Work out the finished part from the listing and answer in its coordinate system (mm). A direction names the side the tool comes from. Give positions to 0.01 mm unless a question says otherwise; leave off trailing zeros. Loops run counter-clockwise (first coordinate to the right, second up) from the corner with the lowest first, then second, coordinate; pieces in that order, holes last. Notation, with made-up numbers: M 15.5,-10.75 L 51.5,-10.75 A33 ccw 51.5,26.25 Z; hole C 29,64 d10. An arc over 180 degrees is marked long. Use a Markdown table: item, result.
```python
from build123d import *

# Parameters (mm, degrees)
SKETCH1_R                                    = 65
BOSS_EXTRUDE2_DEPTH                          = 30
SKETCH2_R                                    = 52.6
CUT_EXTRUDE1_DEPTH                           = 84
SKETCH4_R                                    = 52.6
BOSS_EXTRUDE3_DEPTH                          = 5
SKETCH5_W                                    = 16.2
SKETCH5_H                                    = 9.2
CUT_EXTRUDE2_DEPTH                           = 12
CUT_EXTRUDE3_DEPTH                           = 5.2
M6_CLEARANCE_HOLE1_D                         = 7
CUT_EXTRUDE4_START                           = -18
SKETCH11_R                                   = 65
CUT_EXTRUDE4_DEPTH                           = 18
SKETCH12_R                                   = 65
BOSS_EXTRUDE4_DEPTH                          = 5
CSK_FOR_M6_COUNTERSUNK_FLAT_HEAD_SCR_2_COUNT = 2
CSK_FOR_M6_COUNTERSUNK_FLAT_HEAD_SCR_2_PITCH = 35.355339059
CSK_FOR_M6_COUNTERSUNK_FLAT_HEAD_SCR_3_COUNT = 2
CSK_FOR_M6_COUNTERSUNK_FLAT_HEAD_SCR_3_PITCH = 50
CSK_FOR_M6_COUNTERSUNK_FLAT_HEAD_SCR_4_COUNT = 2
CSK_FOR_M6_COUNTERSUNK_FLAT_HEAD_SCR_4_PITCH = 50
CSK_FOR_M6_COUNTERSUNK_FLAT_HEAD_SCR_5_COUNT = 2
CSK_FOR_M6_COUNTERSUNK_FLAT_HEAD_SCR_5_PITCH = 35.355339059
CSK_FOR_M6_COUNTERSUNK_FLAT_HEAD_SCR_6_COUNT = 2
CSK_FOR_M6_COUNTERSUNK_FLAT_HEAD_SCR_6_PITCH = 35.355339059
CUT_EXTRUDE5_START                           = -3
SKETCH22_R                                   = 65
CUT_EXTRUDE5_DEPTH                           = 3


with BuildPart() as part:
    # Sketch1 → Boss-Extrude2 (new body)
    with BuildSketch(Plane(origin=(0, 0, 0), x_dir=(1, 0, 0), z_dir=(0, 1, 0))):
        with Locations(Location((0, 0, 0), (0, 0, 270))):
            Circle(SKETCH1_R)
    extrude(amount=BOSS_EXTRUDE2_DEPTH)

    # Sketch2 → Cut-Extrude1 (cut)
    with BuildSketch(Plane(origin=(0, 30, 0), x_dir=(1, 0, 0), z_dir=(0, 1, 0))):
        with Locations(Location((0, 0, 0), (0, 0, 270))):
            Circle(SKETCH2_R)
    extrude(amount=-CUT_EXTRUDE1_DEPTH, mode=Mode.SUBTRACT)

    # Sketch4 → Boss-Extrude3 (add)
    with BuildSketch(Plane(origin=(0, 30, 0), x_dir=(1, 0, 0), z_dir=(0, 1, 0))):
        with Locations(Location((0, 0, 0), (0, 0, 270))):
            Circle(SKETCH4_R)
    extrude(amount=-BOSS_EXTRUDE3_DEPTH)

    # Sketch5 → Cut-Extrude2 (cut)
    with BuildSketch(Plane.XZ):
        with Locations((-52.6, 0)):
            Rectangle(SKETCH5_W, SKETCH5_H)
        with Locations((52.6, 0)):
            Rectangle(SKETCH5_W, SKETCH5_H)
    extrude(amount=-CUT_EXTRUDE2_DEPTH, mode=Mode.SUBTRACT)

    # Sketch7 → Cut-Extrude3 (cut)
    with BuildSketch(Plane.XZ.offset(-12)):
        with BuildLine():
            Line((37.19381669, -37.19381669), (44.070308528, -44.070308528))
            ThreePointArc((44.070308528, -44.070308528), (57.580632973, -23.850679107), (62.324828018, 0))
            Line((62.324828018, 0), (52.6, 0))
            ThreePointArc((52.6, 0), (48.59606341, -20.129148542), (37.19381669, -37.19381669))
        make_face()
        with BuildLine():
            Line((-37.19381669, 37.19381669), (-44.070308528, 44.070308528))
            ThreePointArc((-44.070308528, 44.070308528), (-57.580632973, 23.850679107), (-62.324828018, 0))
            Line((-62.324828018, 0), (-52.6, 0))
            ThreePointArc((-52.6, 0), (-48.59606341, 20.129148542), (-37.19381669, 37.19381669))
        make_face()
    extrude(amount=CUT_EXTRUDE3_DEPTH, mode=Mode.SUBTRACT)

    # M6 Clearance Hole1 (through all)
    with Locations(Plane(origin=(0, 30, -25), x_dir=(0, 0, 1), z_dir=(0, 1, 0))):
        with Locations((0, 0), (25, -25), (25, 25), (50, 0)):
            Hole(M6_CLEARANCE_HOLE1_D / 2)

    # Sketch11 → Cut-Extrude4 (cut)
    with BuildSketch(Plane(origin=(0, 30, 0), x_dir=(1, 0, 0), z_dir=(0, 1, 0)).offset(CUT_EXTRUDE4_START)):
        with Locations(Location((0, 0, 0), (0, 0, 270))):
            Circle(SKETCH11_R)
    extrude(amount=CUT_EXTRUDE4_DEPTH, mode=Mode.SUBTRACT)

    # Sketch12 → Boss-Extrude4 (add)
    with BuildSketch(Plane(origin=(0, 12, 0), x_dir=(1, 0, 0), z_dir=(0, 1, 0))):
        with Locations(Location((0, 0, 0), (0, 0, 270))):
            Circle(SKETCH12_R)
    extrude(amount=BOSS_EXTRUDE4_DEPTH)

    # Sketch21 → CSK for M6 Countersunk Flat Head Screw3 (revolve, cut)
    with BuildSketch(Plane(origin=(25, 12, 0), x_dir=(0, 0, -1), z_dir=(1, 0, 0))):
        Polygon((0, 0), (0, 5), (3.5, 5), (3.5, 2.8), (6.3, 0), align=None)
    csk_for_m6_countersunk_flat_head_screw3 = revolve(axis=Axis((25, 5.65, 0), (0, 1, 0)), mode=Mode.SUBTRACT)

    # CSK for M6 Countersunk Flat Head Scr 2: CSK for M6 Countersunk Flat Head Screw3 ×2
    with Locations(*[Vector(-0.7071067811865476, 0, 0.7071067811865476) * (i * CSK_FOR_M6_COUNTERSUNK_FLAT_HEAD_SCR_2_PITCH) for i in range(1, CSK_FOR_M6_COUNTERSUNK_FLAT_HEAD_SCR_2_COUNT)]):
        add(csk_for_m6_countersunk_flat_head_screw3, mode=Mode.SUBTRACT)

    # CSK for M6 Countersunk Flat Head Scr 3: CSK for M6 Countersunk Flat Head Screw3 ×2
    with Locations(*[(-i * CSK_FOR_M6_COUNTERSUNK_FLAT_HEAD_SCR_3_PITCH, 0, 0) for i in range(1, CSK_FOR_M6_COUNTERSUNK_FLAT_HEAD_SCR_3_COUNT)]):
        add(csk_for_m6_countersunk_flat_head_screw3, mode=Mode.SUBTRACT)

    # CSK for M6 Countersunk Flat Head Scr 4: CSK for M6 Countersunk Flat Head Screw3 ×2
    with Locations(*[(-i * CSK_FOR_M6_COUNTERSUNK_FLAT_HEAD_SCR_4_PITCH, 0, 0) for i in range(1, CSK_FOR_M6_COUNTERSUNK_FLAT_HEAD_SCR_4_COUNT)]):
        add(csk_for_m6_countersunk_flat_head_screw3, mode=Mode.SUBTRACT)

    # CSK for M6 Countersunk Flat Head Scr 5: CSK for M6 Countersunk Flat Head Screw3 ×2
    with Locations(*[Vector(-0.7071067811865476, 0, 0.7071067811865476) * (i * CSK_FOR_M6_COUNTERSUNK_FLAT_HEAD_SCR_5_PITCH) for i in range(1, CSK_FOR_M6_COUNTERSUNK_FLAT_HEAD_SCR_5_COUNT)]):
        add(csk_for_m6_countersunk_flat_head_screw3, mode=Mode.SUBTRACT)

    # CSK for M6 Countersunk Flat Head Scr 6: CSK for M6 Countersunk Flat Head Screw3 ×2
    with Locations(*[Vector(-0.7071067811865476, 0, -0.7071067811865476) * (i * CSK_FOR_M6_COUNTERSUNK_FLAT_HEAD_SCR_6_PITCH) for i in range(1, CSK_FOR_M6_COUNTERSUNK_FLAT_HEAD_SCR_6_COUNT)]):
        add(csk_for_m6_countersunk_flat_head_screw3, mode=Mode.SUBTRACT)

    # Sketch22 → Cut-Extrude5 (cut)
    with BuildSketch(Plane.XZ.offset(CUT_EXTRUDE5_START)):
        with Locations(Location((0, 0, 0), (0, 0, 270))):
            Circle(SKETCH22_R)
        with BuildLine():
            Line((-52.39847326, 4.6), (-60.7, 4.6))
            Line((-60.7, 4.6), (-60.7, -4.6))
            Line((-60.7, -4.6), (-52.39847326, -4.6))
            ThreePointArc((-52.39847326, -4.6), (0, -52.6), (52.39847326, -4.6))
            Line((52.39847326, -4.6), (60.7, -4.6))
            Line((60.7, -4.6), (60.7, 4.6))
            Line((60.7, 4.6), (52.39847326, 4.6))
            ThreePointArc((52.39847326, 4.6), (0, 52.6), (-52.39847326, 4.6))
        make_face(mode=Mode.SUBTRACT)
    extrude(amount=CUT_EXTRUDE5_DEPTH, mode=Mode.SUBTRACT)


solid = part.part
```
(1) Which of the six approach directions +Z, -Z, +X, -X, +Y, -Y give full straight-line access (tool end or side, diameter ignored) to faces 1 (the flat face through (56, 5, -4.6)), 2 (the flat face through (41, 9, -41)), 3 (the flat face through (1, 17, -1))?
Entries:
| item | result |
|---|---|
| face 1 | -Y |
| face 2 | none |
| face 3 | +Z, -Z, +X, -X, +Y |
(2) A cutting plane is placed at B-B (z = -25). Write down the section's boundary in (x, y), and give its area (3 significant figures).
Entries:
| item | result |
|---|---|
| outline | M -60,3 L -46.28,3 L -46.28,12 L -6.3,12 L -3.5,14.8 L -3.5,17 L -60,17 Z; M 3.5,14.8 L 6.3,12 L 57.09,12 L 57.09,6.8 L 46.28,6.8 L 46.28,3 L 60,3 L 60,17 L 3.5,17 Z |
| area | 748 mm² |
(3) A cutting plane is placed at D-D (z = 12.5). Write down the section's boundary in (x, y).
Entries:
| item | result |
|---|---|
| outline | M -63.79,3 L -51.09,3 L -51.09,6.8 L -61.06,6.8 L -61.06,12 L 51.09,12 L 51.09,3 L 63.79,3 L 63.79,17 L -63.79,17 Z |
(4) Given P1, Ø3, axis at x = -6, z = 46, coming from the -Y side; P2, Ø1.9, axis at x = -58.5, y = 4.5, coming from the -Z side; P3, Ø3, axis at x = 57.5, y = 4.5, coming from the +Z side; P4, Ø5.5, axis at x = -25, z = 0, coming from the +Y side, each flat-ended and moving along its own axis, determine where each tip first touches the part or whether it passes through.
Entries:
| item | result |
|---|---|
| P1 | stops at y = 12 |
| P2 | stops at z = -30.22 |
| P3 | stops at z = 33 |
| P4 | passes through |
(5) A cutting plane is placed at A-A (x = 0). Write down the section's boundary in (y, z).
Entries:
| item | result |
|---|---|
| outline | M 3,-65 L 17,-65 L 17,-28.5 L 14.8,-28.5 L 12,-31.3 L 12,-52.6 L 3,-52.6 Z; M 3,52.6 L 12,52.6 L 12,31.3 L 14.8,28.5 L 17,28.5 L 17,65 L 3,65 Z; M 12,-18.7 L 14.8,-21.5 L 17,-21.5 L 17,21.5 L 14.8,21.5 L 12,18.7 Z |
(6) The mould has two halves that part along Z. Classify faces 4 (the cylindrical face through (19.52, 9.9, 62)), 5 (the cylindrical face through (-28.47, 15.88, 0.46)), 6 (the flat face through (53, 3, 5)): released by +Z, released by -Z, zero draft, split by the parting line, or undercut.
Entries:
| item | result |
|---|---|
| face 4 | split by the parting line |
| face 5 | undercut |
| face 6 | zero draft |
(7) A cutting plane is placed at C-C (x = 25). Write down the section's boundary in (y, z).
Entries:
| item | result |
|---|---|
| outline | M 3,-60 L 17,-60 L 17,-3.5 L 14.8,-3.5 L 12,-6.3 L 12,-46.28 L 3,-46.28 Z; M 3,46.28 L 12,46.28 L 12,6.3 L 14.8,3.5 L 17,3.5 L 17,60 L 3,60 Z |
(8) Consider probe 1 along X at (y, z) = (16.1, 0); probe 2 along Y at (x, z) = (43, 14.5); probe 3 along X at (y, z) = (7, 13). Determine where each line is inside the solid, lowest interval first. Write a range as [from, to].
Entries:
| item | result |
|---|---|
| probe 1 | x = [-65, -28.5], [-21.5, 21.5], [28.5, 65] |
| probe 2 | y = [12, 17] |
| probe 3 | x = [-63.69, -60.95], [50.97, 63.69] |
